The listing builds one solid part. Answer for the finished solid, in the listing's coordinates (mm). A direction names the side the tool comes from. Give positions to 0.01 mm unless a question says otherwise; leave off trailing zeros. Write each loop counter-clockwise with the first axis right and the second up, starting at its lowest first coordinate (ties: lowest second). Pieces come first, ordered by that corner, then holes. Notation, with made-up numbers: (-28, 26.25) -> (21, 26.25) arc R15 cw to (21, 47.25) -> close; hole circle Ø10 at (-4, 46.5). An arc over 180 degrees is marked (long way). One line per question, with ' | ' between items.
from build123d import *

# Parameters (mm, degrees)
BOSS_EXTRUDE1_DEPTH = 15
CUT_EXTRUDE1_DEPTH  = 7.5
SKETCH3_R           = 6.92
CUT_EXTRUDE2_DEPTH  = 7.5
SKETCH4_R           = 5
CUT_EXTRUDE3_DEPTH  = 15
THREAD1_PITCH       = 1.5


with BuildPart() as part:
    # Sketch1 → Boss-Extrude1 (new body)
    with BuildSketch(Plane(origin=(0, 0, 0), x_dir=(1, 0, 0), z_dir=(0, 1, 0))):
        with BuildLine():
            Line((-100, -120), (-100, 120))
            ThreePointArc((-100, 120), (-88.284271247, 148.284271247), (-60, 160))
            Line((-60, 160), (60, 160))
            ThreePointArc((60, 160), (88.284271247, 148.284271247), (100, 120))
            Line((100, 120), (100, -120))
            ThreePointArc((100, -120), (88.284271247, -148.284271247), (60, -160))
            Line((60, -160), (-60, -160))
            ThreePointArc((-60, -160), (-88.284271247, -148.284271247), (-100, -120))
        make_face()
    extrude(amount=BOSS_EXTRUDE1_DEPTH)

    # Sketch2 → Cut-Extrude1 (cut)
    with BuildSketch(Plane.XZ):
        with BuildLine():
            Line((80, -120), (80, 120))
            ThreePointArc((80, 120), (74.142135624, 134.142135624), (60, 140))
            Line((60, 140), (-60, 140))
            ThreePointArc((-60, 140), (-74.142135624, 134.142135624), (-80, 120))
            Line((-80, 120), (-80, -120))
            ThreePointArc((-80, -120), (-74.142135624, -134.142135624), (-60, -140))
            Line((-60, -140), (60, -140))
            ThreePointArc((60, -140), (74.142135624, -134.142135624), (80, -120))
        make_face()
    extrude(amount=-CUT_EXTRUDE1_DEPTH, mode=Mode.SUBTRACT)

    # Sketch3 → Cut-Extrude2 (cut)
    with BuildSketch(Plane.XZ.offset(-7.5)):
        with Locations(Location((0, 0, 0), (0, 0, 270))):
            Circle(SKETCH3_R)
    extrude(amount=-CUT_EXTRUDE2_DEPTH, mode=Mode.SUBTRACT)

    # Sketch4 → Cut-Extrude3 (cut)
    with BuildSketch(Plane.XZ):
        with Locations(Location((40, 150, 0), (0, 0, 270))):
            Circle(SKETCH4_R)
        with Locations(Location((90, 0, 0), (0, 0, 270))):
            Circle(SKETCH4_R)
        with Locations(Location((90, 100, 0), (0, 0, 270))):
            Circle(SKETCH4_R)
        with Locations(Location((90, -100, 0), (0, 0, 270))):
            Circle(SKETCH4_R)
        with Locations(Location((40, -150, 0), (0, 0, 270))):
            Circle(SKETCH4_R)
        with Locations(Location((-40, -150, 0), (0, 0, 270))):
            Circle(SKETCH4_R)
        with Locations(Location((-90, -100, 0), (0, 0, 270))):
            Circle(SKETCH4_R)
        with Locations(Location((-90, 100, 0), (0, 0, 270))):
            Circle(SKETCH4_R)
        with Locations(Location((-90, 0, 0), (0, 0, 270))):
            Circle(SKETCH4_R)
        with Locations(Location((-40, 150, 0), (0, 0, 270))):
            Circle(SKETCH4_R)
    extrude(amount=-CUT_EXTRUDE3_DEPTH, mode=Mode.SUBTRACT)

    # Thread1: the profile of Thread Profile1 profile screwed along a right-hand helix of 5 turns, 8 arcs to a turn; built about Z, then put on its axis
    thread1_z = Axis((0, 0, 0), (0, 0, 1))
    thread1_corners = [(6.9197, 0, -0.000173205), (7.731898812, 0, 0.468749998), (7.731898812, 0, 0.656249998), (6.9197, 0, 1.125173201)]
    with BuildLine(mode=Mode.PRIVATE) as thread1_profile:
        Line(thread1_corners[0], thread1_corners[1])
        Line(thread1_corners[1], thread1_corners[2])
        Line(thread1_corners[2], thread1_corners[3])
        Line(thread1_corners[3], thread1_corners[0])
    thread1_cap = Face(thread1_profile.wire())
    thread1_turn_angles = [0, 22.5, 45, 67.5, 90, 112.5, 135, 157.5, 180, 202.5, 225, 247.5, 270, 292.5, 315, 337.5, 360]
    thread1_turn_weights = [1, 0.9238795325112867, 1, 0.9238795325112867, 1, 0.9238795325112867, 1, 0.9238795325112867, 1, 0.9238795325112867, 1, 0.9238795325112867, 1, 0.9238795325112867, 1, 0.9238795325112867, 1]
    thread1_turn_rails = [Edge.make_bspline([Vector(p[0], p[1], 0).rotate(thread1_z, thread1_turn_angles[k]) / thread1_turn_weights[k] + Vector(0, 0, p[2] + THREAD1_PITCH * thread1_turn_angles[k] / 360) for k in range(17)], [0, 0, 0, 1, 1, 2, 2, 3, 3, 4, 4, 5, 5, 6, 6, 7, 7, 8, 8, 8], 2, thread1_turn_weights) for p in thread1_corners]
    thread1_turn_sides = [Face.make_surface_from_curves(thread1_turn_rails[p[0]], thread1_turn_rails[p[1]]) for p in [(0, 1), (1, 2), (2, 3), (3, 0)]]
    thread1 = Plane(origin=(0, 7.5, 0), x_dir=(1, 0, 0), z_dir=(0, 1, 0)) * Solid(Shell([*[p.moved(Location((0, 0, THREAD1_PITCH * i))) for i in range(5) for p in thread1_turn_sides], thread1_cap, thread1_cap.rotate(thread1_z, 1800).moved(Location((0, 0, THREAD1_PITCH * 1800 / 360)))]))
    add(thread1, mode=Mode.SUBTRACT)


solid = part.part
Item 1: Determine the mould class of faces 3 (the face through (88.085, 7.395, -104.619)), 4 (the face through (1, 7, 160)), 5 (the face through (-1, 7, -160)) for opening direction Z: pulls with the +Z half, pulls with the -Z half, needs draft (parallel to the pull), parting line crosses it, or undercut.
Answers below:
face 3: undercut | face 4: pulls with the +Z half | face 5: pulls with the -Z half
Item 2: Find section C-C (x = -90). Write down the section's boundary in (y, z).
Answers below:
outline: (0, -146.46) -> (15, -146.46) -> (15, -105) -> (0, -105) -> close; (0, -95) -> (15, -95) -> (15, -5) -> (0, -5) -> close; (0, 5) -> (15, 5) -> (15, 95) -> (0, 95) -> close; (0, 105) -> (15, 105) -> (15, 146.46) -> (0, 146.46) -> close
Item 3: Find section D-D (z = -150). Write down the section's boundary in (x, y).
Answers below:
outline: (-86.46, 0) -> (-45, 0) -> (-45, 15) -> (-86.46, 15) -> close; (-35, 0) -> (35, 0) -> (35, 15) -> (-35, 15) -> close; (45, 0) -> (86.46, 0) -> (86.46, 15) -> (45, 15) -> close
Item 4: Consider line 1 (X direction, y = 3.75, z = 0); line 2 (X direction, y = 9.25, z = 100); line 3 (X direction, y = 6.5, z = 102). Determine where each line is inside the solid, lowest interval first. Write a range as [from, to].
Answers below:
line 1: [-100, -95], [-85, -80], [80, 85], [95, 100] | line 2: [-100, -95], [-85, 85], [95, 100] | line 3: [-100, -94.58], [-85.42, -80], [80, 85.42], [94.58, 100]
Item 5: Flat-ended cylindrical pins translate along their axes: pin 1 (1 mm diameter, centred on x = 66.5, y = 8, fed in from +Z); pin 2 (12 mm diameter, centred on x = -44.5, z = -56.5, fed in from -Y). Find the tip coordinate at first contact, or state that the pin passes through.
Answers below:
pin 1: z = 159.55 | pin 2: y = 7.5
Item 6: A tool of negligible diameter and unlimited length cuts with its end or side. For faces 1 (the face through (-91.915, 7.395, 95.381)), 2 (the face through (74.297, 3.698, 133.986)), from which of +Z, -Z, +X, -X, +Y, -Y can it reach the whole face along a straight path? Write none if from no direction.
Answers below:
face 1: +Y, -Y | face 2: -Y
Item 7: Find section A-A (x = 40). Write down the section's boundary in (y, z), then the cut area to 3 significant figures.
Answers below:
outline: (0, -160) -> (15, -160) -> (15, -155) -> (0, -155) -> close; (0, -145) -> (15, -145) -> (15, 145) -> (0, 145) -> (0, 140) -> (7.5, 140) -> (7.5, -140) -> (0, -140) -> close; (0, 155) -> (15, 155) -> (15, 160) -> (0, 160) -> close | area: 2,400 mm²
Item 8: Find section B-B (y = 3). Count the separate pieces of the cut face and the enclosed holes in it, then the cut area to 3 significant figures.
Answers below:
separate pieces: 1 | enclosed holes: 11 | area: 17,400 mm²
